```python
from build123d import *

# Parameters (mm, degrees)
SKETCH1_R           = 75
SKETCH1_R_2         = 30
BOSS_EXTRUDE1_DEPTH = 5
CUT_EXTRUDE1_DEPTH  = 107.183802908


with BuildPart() as part:
    # Sketch1 → Boss-Extrude1 (new body)
    with BuildSketch(Plane(origin=(0, 0, 0), x_dir=(1, 0, 0), z_dir=(0, 1, 0))):
        with Locations(Location((0, 0, 0), (0, 0, 270))):
            Circle(SKETCH1_R)
        with Locations(Location((0, 0, 0), (0, 0, 270))):
            Circle(SKETCH1_R_2, mode=Mode.SUBTRACT)
        with BuildLine():
            Line((-5, 41.802033443), (-5, 37.568737003))
            ThreePointArc((-5, 37.568737003), (-26.799347007, 26.799347007), (-37.568737003, 5))
            Line((-37.568737003, 5), (-41.802033443, 5))
            ThreePointArc((-41.802033443, 5), (-29.769195488, 29.769195488), (-5, 41.802033443))
        make_face(mode=Mode.SUBTRACT)
        with BuildLine():
            Line((5, 41.802033443), (5, 37.568737003))
            ThreePointArc((5, 37.568737003), (26.799347007, 26.799347007), (37.568737003, 5))
            Line((37.568737003, 5), (41.802033443, 5))
            ThreePointArc((41.802033443, 5), (29.769195488, 29.769195488), (5, 41.802033443))
        make_face(mode=Mode.SUBTRACT)
        with BuildLine():
            Line((41.802033443, -5), (37.568737003, -5))
            ThreePointArc((37.568737003, -5), (26.799347007, -26.799347007), (5, -37.568737003))
            Line((5, -37.568737003), (5, -41.802033443))
            ThreePointArc((5, -41.802033443), (29.769195488, -29.769195488), (41.802033443, -5))
        make_face(mode=Mode.SUBTRACT)
        with BuildLine():
            Line((-5, -41.802033443), (-5, -37.568737003))
            ThreePointArc((-5, -37.568737003), (-26.799347007, -26.799347007), (-37.568737003, -5))
            Line((-37.568737003, -5), (-41.802033443, -5))
            ThreePointArc((-41.802033443, -5), (-29.769195488, -29.769195488), (-5, -41.802033443))
        make_face(mode=Mode.SUBTRACT)
    extrude(amount=BOSS_EXTRUDE1_DEPTH)

    # Sketch4 → Cut-Extrude1 (cut, through all)
    with BuildSketch(Plane(origin=(0, 5, 0), x_dir=(1, 0, 0), z_dir=(0, 1, 0))):
        with BuildLine():
            Line((-6.5, 51), (-6.5, 66))
            ThreePointArc((-6.5, 66), (0, 72.5), (6.5, 66))
            Line((6.5, 66), (6.5, 51))
            ThreePointArc((6.5, 51), (0, 44.5), (-6.5, 51))
        make_face()
        with BuildLine():
            Line((31.129165125, 40.917295593), (38.629165125, 53.90767665))
            ThreePointArc((38.629165125, 53.90767665), (36.25, 62.786841774), (27.370834875, 60.40767665))
            Line((27.370834875, 60.40767665), (19.870834875, 47.417295593))
            ThreePointArc((19.870834875, 47.417295593), (22.25, 38.538130468), (31.129165125, 40.917295593))
        make_face()
        with BuildLine():
            Line((47.417295593, 19.870834875), (60.40767665, 27.370834875))
            ThreePointArc((60.40767665, 27.370834875), (62.786841774, 36.25), (53.90767665, 38.629165125))
            Line((53.90767665, 38.629165125), (40.917295593, 31.129165125))
            ThreePointArc((40.917295593, 31.129165125), (38.538130468, 22.25), (47.417295593, 19.870834875))
        make_face()
        with BuildLine():
            Line((51, -6.5), (66, -6.5))
            ThreePointArc((66, -6.5), (72.5, 0), (66, 6.5))
            Line((66, 6.5), (51, 6.5))
            ThreePointArc((51, 6.5), (44.5, 0), (51, -6.5))
        make_face()
        with BuildLine():
            Line((40.917295593, -31.129165125), (53.90767665, -38.629165125))
            ThreePointArc((53.90767665, -38.629165125), (62.786841774, -36.25), (60.40767665, -27.370834875))
            Line((60.40767665, -27.370834875), (47.417295593, -19.870834875))
            ThreePointArc((47.417295593, -19.870834875), (38.538130468, -22.25), (40.917295593, -31.129165125))
        make_face()
        with BuildLine():
            Line((19.870834875, -47.417295593), (27.370834875, -60.40767665))
            ThreePointArc((27.370834875, -60.40767665), (36.25, -62.786841774), (38.629165125, -53.90767665))
            Line((38.629165125, -53.90767665), (31.129165125, -40.917295593))
            ThreePointArc((31.129165125, -40.917295593), (22.25, -38.538130468), (19.870834875, -47.417295593))
        make_face()
        with BuildLine():
            Line((-6.5, -51), (-6.5, -66))
            ThreePointArc((-6.5, -66), (0, -72.5), (6.5, -66))
            Line((6.5, -66), (6.5, -51))
            ThreePointArc((6.5, -51), (0, -44.5), (-6.5, -51))
        make_face()
        with BuildLine():
            Line((-31.129165125, -40.917295593), (-38.629165125, -53.90767665))
            ThreePointArc((-38.629165125, -53.90767665), (-36.25, -62.786841774), (-27.370834875, -60.40767665))
            Line((-27.370834875, -60.40767665), (-19.870834875, -47.417295593))
            ThreePointArc((-19.870834875, -47.417295593), (-22.25, -38.538130468), (-31.129165125, -40.917295593))
        make_face()
        with BuildLine():
            Line((-47.417295593, -19.870834875), (-60.40767665, -27.370834875))
            ThreePointArc((-60.40767665, -27.370834875), (-62.786841774, -36.25), (-53.90767665, -38.629165125))
            Line((-53.90767665, -38.629165125), (-40.917295593, -31.129165125))
            ThreePointArc((-40.917295593, -31.129165125), (-38.538130468, -22.25), (-47.417295593, -19.870834875))
        make_face()
        with BuildLine():
            Line((-51, 6.5), (-66, 6.5))
            ThreePointArc((-66, 6.5), (-72.5, 0), (-66, -6.5))
            Line((-66, -6.5), (-51, -6.5))
            ThreePointArc((-51, -6.5), (-44.5, 0), (-51, 6.5))
        make_face()
        with BuildLine():
            Line((-40.917295593, 31.129165125), (-53.90767665, 38.629165125))
            ThreePointArc((-53.90767665, 38.629165125), (-62.786841774, 36.25), (-60.40767665, 27.370834875))
            Line((-60.40767665, 27.370834875), (-47.417295593, 19.870834875))
            ThreePointArc((-47.417295593, 19.870834875), (-38.538130468, 22.25), (-40.917295593, 31.129165125))
        make_face()
        with BuildLine():
            Line((-19.870834875, 47.417295593), (-27.370834875, 60.40767665))
            ThreePointArc((-27.370834875, 60.40767665), (-36.25, 62.786841774), (-38.629165125, 53.90767665))
            Line((-38.629165125, 53.90767665), (-31.129165125, 40.917295593))
            ThreePointArc((-31.129165125, 40.917295593), (-22.25, 38.538130468), (-19.870834875, 47.417295593))
        make_face()
    extrude(amount=-CUT_EXTRUDE1_DEPTH, mode=Mode.SUBTRACT)


solid = part.part
```
For this review, take the finished solid that the model builds, in its own axes (mm). Round coordinates to 2 decimals unless told otherwise and drop trailing zeros. Write each loop counter-clockwise with the first axis right and the second up, starting at its lowest first coordinate (ties: lowest second). Pieces come first, ordered by that corner, then holes. Notation, with made-up numbers: (87.5, -32.75) - (135.5, -32.75) arc R27 cw to (135.5, -16.75) - close; hole circle Ø2 at (-37.75, 54.5). An arc over 180 degrees is marked (long way). Answer as a JSON object with one key per item and string values.
1. We need section A-A on x = 0. Give the boundary of the cut face in (y, z).
Response values:
{"outline": "(0, -75) - (5, -75) - (5, -72.5) - (0, -72.5) - close; (0, -44.5) - (5, -44.5) - (5, -30) - (0, -30) - close; (0, 30) - (5, 30) - (5, 44.5) - (0, 44.5) - close; (0, 72.5) - (5, 72.5) - (5, 75) - (0, 75) - close"}
2. We need section D-D on z = -33. Give the boundary of the cut face in (x, y), then the cut area to 3 significant figures.
Response values:
{"outline": "(-67.35, 0) - (-63.66, 0) - (-63.66, 5) - (-67.35, 5) - close; (-44.16, 0) - (-26.14, 0) - (-26.14, 5) - (-44.16, 5) - close; (-18.64, 0) - (18.64, 0) - (18.64, 5) - (-18.64, 5) - close; (26.14, 0) - (44.16, 0) - (44.16, 5) - (26.14, 5) - close; (63.66, 0) - (67.35, 0) - (67.35, 5) - (63.66, 5) - close", "area": "403 mm2"}
3. To check wall thickness, follow line 1 along X through (y, z) = (2.4, 0); line 2 along X through (y, z) = (4.2, -56); line 3 along X through (y, z) = (4.8, 5.5). State the ranges of each line that lie inside material, in increasing order.
Response values:
{"line 1": "x = -75 to -72.5, -44.5 to -30, 30 to 44.5, 72.5 to 75", "line 2": "x = -49.89 to -39.4, -24.83 to -6.5, 6.5 to 24.83, 39.4 to 49.89", "line 3": "x = -74.8 to -69.46, -47.54 to -41.74, -37.5 to -29.49, 29.49 to 37.5, 41.74 to 47.54, 69.46 to 74.8"}
4. We need section C-C on x = -23. Give the boundary of the cut face in (y, z), then the cut area to 3 significant figures.
Response values:
{"outline": "(0, -71.39) - (5, -71.39) - (5, -52.84) - (0, -52.84) - close; (0, -38.17) - (5, -38.17) - (5, -35.26) - (0, -35.26) - close; (0, -30.12) - (5, -30.12) - (5, -19.26) - (0, -19.26) - close; (0, 19.26) - (5, 19.26) - (5, 30.12) - (0, 30.12) - close; (0, 35.26) - (5, 35.26) - (5, 38.17) - (0, 38.17) - close; (0, 52.84) - (5, 52.84) - (5, 71.39) - (0, 71.39) - close", "area": "323 mm2"}
5. Draft analysis for pull direction X (two halves, no side actions). For faces 1 (the face through (-54, 2.54, -23.67)), 2 (the face through (-32, 0, -1)), state which applies: +X half, -X half, draft (parallel to the pull), parting line (faces both ways), or undercut.
Response values:
{"face 1": "undercut", "face 2": "draft"}
6. We need section B-B on z = -17. Give the boundary of the cut face in (x, y).
Response values:
{"outline": "(-73.05, 0) - (-38.52, 0) - (-38.52, 5) - (-73.05, 5) - close; (-33.87, 0) - (-24.72, 0) - (-24.72, 5) - (-33.87, 5) - close; (24.72, 0) - (33.87, 0) - (33.87, 5) - (24.72, 5) - close; (38.52, 0) - (73.05, 0) - (73.05, 5) - (38.52, 5) - close"}
7. For pin 1 Ø2.5 at (y, z) = (3.5, 58) entering from -X; pin 2 Ø3 at (x, y) = (18, 1.5) entering from +Z; pin 3 Ø2.5 at (x, y) = (61, 1.5) entering from +Z, all flat-tipped, find the tip position at first contact; note any pin that passes through.
Response values:
{"pin 1": "stops at x = -49.04", "pin 2": "stops at z = 73.16", "pin 3": "stops at z = 45.33"}
